Could you check a few things on this drawing? It's one solid part, dimensions in mm from its lowest x, y, z. A direction names the side the tool comes from. Round coordinates to 2 decimals unless told otherwise and drop trailing zeros. Loops run counter-clockwise (first coordinate to the right, second up) from the corner with the lowest first, then second, coordinate; pieces in that order, holes last. Notation, with made-up numbers: M 54,37 L 96,37 A19 ccw 96,51 Z; hole C 31.5,44 d9. An arc over 180 degrees is marked long. Return JSON: item names as keys, results as strings.
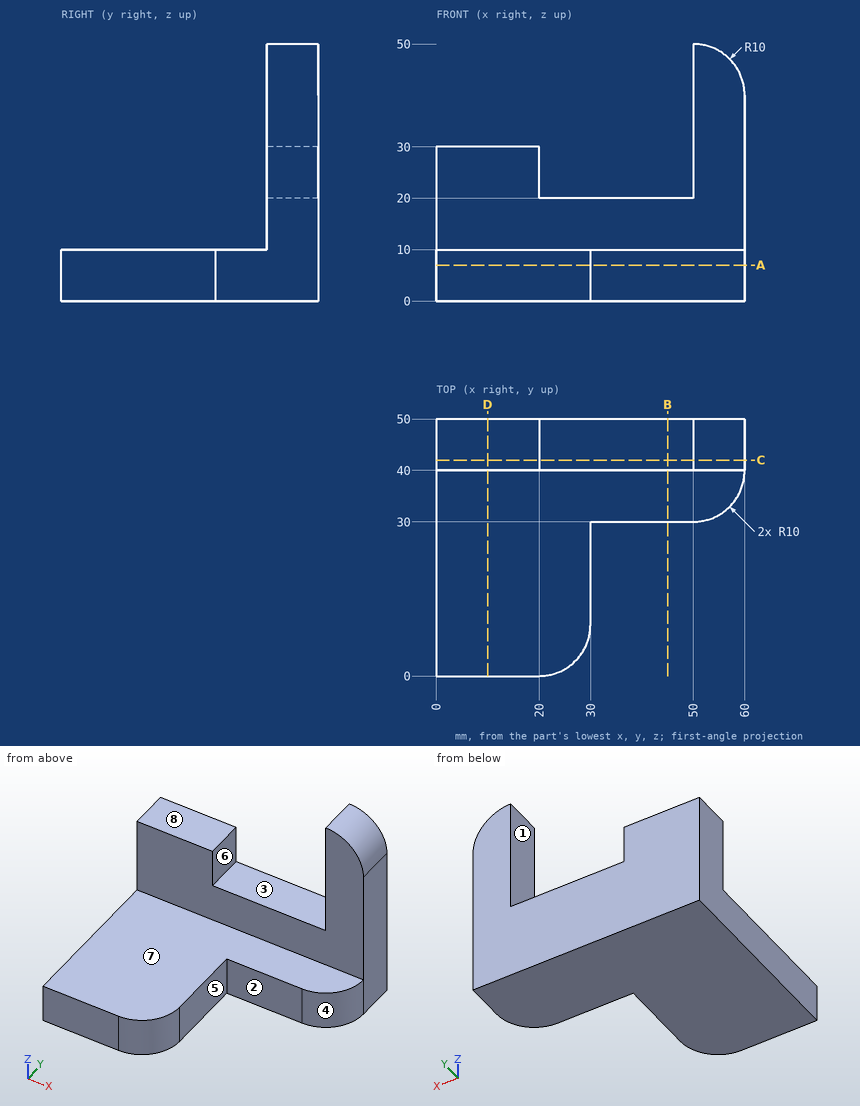
Q1. Suppose I cut it at D-D, the plane x = 10. Please give me the cut outline in (y, z), plus the area to 3 significant figures.
Results:
{"outline": "M 0,0 L 50,0 L 50,30 L 40,30 L 40,10 L 0,10 Z", "area": "700 mm2"}
Q2. If I drill on line 1 along X through (y, z) = (43, 29); line 2 along Z through (x, y) = (14, 45.5); line 3 along Z through (x, y) = (27, 30), over which ranges is the centre line in solid material (lowest first)?
Results:
{"line 1": "x = 0 to 20, 50 to 60", "line 2": "z = 0 to 30", "line 3": "z = 0 to 10"}
Q3. Suppose I cut it at A-A, the plane z = 7. Please give me the cut outline in (x, y).
Results:
{"outline": "M 0,0 L 20,0 A10 ccw 30,10 L 30,30 L 50,30 A10 ccw 60,40 L 60,50 L 0,50 Z"}
Q4. On a 3-axis mill with a long thin cutter (end or side, diameter ignored), from which of +Z, -Z, +X, -X, +Y, -Y can I reach the whole of each face in a straight line? I mean the marked faces 5, 6, 7 and 8. Say none if no direction works.
Results:
{"face 5": "+Z, -Z, +X, -Y", "face 6": "+Z, +Y, -Y", "face 7": "+Z, +X, -X, -Y", "face 8": "+Z, -X, +Y, -Y"}
Q5. I'm going to push flat-ended pins straight in: pin 1 Ø5 at (x, y) = (9, 46) entering from +Z; pin 2 Ø5 at (y, z) = (24, 3) entering from +X; pin 3 Ø1.5 at (x, y) = (17, 11) entering from +Z; pin 4 Ø12 at (x, z) = (29.5, 36) entering from +Y. Where does each tip first touch, or does it pass through?
Results:
{"pin 1": "stops at z = 30", "pin 2": "stops at x = 30", "pin 3": "stops at z = 10", "pin 4": "passes through"}
Q6. Thinking about a two-plate mould opening in X: for the marked faces 1, 2, 3 and 4, which applies, pulls with the +X half, pulls with the -X half, needs draft (parallel to the pull), parting line crosses it, or undercut?
Results:
{"face 1": "undercut", "face 2": "needs draft", "face 3": "undercut", "face 4": "pulls with the +X half"}
Q7. Suppose I cut it at B-B, the plane x = 45. Please give me the cut outline in (y, z), plus the area to 3 significant figures.
Results:
{"outline": "M 30,0 L 50,0 L 50,20 L 40,20 L 40,10 L 30,10 Z", "area": "300 mm2"}
Q8. Suppose I cut it at C-C, the plane y = 42. Please give me the cut outline in (x, z), plus the area to 3 significant figures.
Results:
{"outline": "M 0,0 L 60,0 L 60,40 A10 ccw 50,50 L 50,20 L 20,20 L 20,30 L 0,30 Z", "area": "1,680 mm2"}
